```python
from build123d import *

# Parameters (mm, degrees)
SKETCH1_W           = 44
SKETCH1_H           = 72
BOSS_EXTRUDE1_DEPTH = 3
SKETCH2_W           = 44
SKETCH2_H           = 72
SKETCH2_W_2         = 40
SKETCH2_H_2         = 68
BOSS_EXTRUDE2_DEPTH = 34
SKETCH3_W           = 68
SKETCH3_H           = 109
SKETCH3_W_2         = 44
SKETCH3_H_2         = 72
BOSS_EXTRUDE3_DEPTH = 3
CHAMFER1_SIZE       = 0.528980942
CHAMFER1_SIZE_2     = 3


with BuildPart() as part:
    # Sketch1 → Boss-Extrude1 (new body)
    with BuildSketch(Plane(origin=(0, 0, 0), x_dir=(1, 0, 0), z_dir=(0, 1, 0))):
        with Locations((22, 36)):
            Rectangle(SKETCH1_W, SKETCH1_H)
    extrude(amount=BOSS_EXTRUDE1_DEPTH)

    # Sketch2 → Boss-Extrude2 (add)
    with BuildSketch(Plane(origin=(0, 3, 0), x_dir=(1, 0, 0), z_dir=(0, 1, 0))):
        with Locations((22, 36)):
            Rectangle(SKETCH2_W, SKETCH2_H)
        with Locations((22, 36)):
            Rectangle(SKETCH2_W_2, SKETCH2_H_2, mode=Mode.SUBTRACT)
    extrude(amount=BOSS_EXTRUDE2_DEPTH)

    # Sketch3 → Boss-Extrude3 (add)
    with BuildSketch(Plane(origin=(0, 24.3, 0), x_dir=(1, 0, 0), z_dir=(0, 1, 0))):
        with Locations((22, 36)):
            Rectangle(SKETCH3_W, SKETCH3_H)
        with Locations((22, 36)):
            Rectangle(SKETCH3_W_2, SKETCH3_H_2, mode=Mode.SUBTRACT)
        with BuildLine():
            Line((20.7, -3.5), (23.3, -3.5))
            ThreePointArc((23.3, -3.5), (25.6, -5.8), (23.3, -8.1))
            Line((23.3, -8.1), (20.7, -8.1))
            ThreePointArc((20.7, -8.1), (18.4, -5.8), (20.7, -3.5))
        make_face(mode=Mode.SUBTRACT)
        with BuildLine():
            Line((20.7, 75.5), (23.3, 75.5))
            ThreePointArc((23.3, 75.5), (25.6, 77.8), (23.3, 80.1))
            Line((23.3, 80.1), (20.7, 80.1))
            ThreePointArc((20.7, 80.1), (18.4, 77.8), (20.7, 75.5))
        make_face(mode=Mode.SUBTRACT)
    extrude(amount=BOSS_EXTRUDE3_DEPTH)

    # Chamfer1
    # the kernel refuses this chamfer: 3, 0.528980942 mm, written as the material it takes off along each edge
    with BuildSketch(Plane(origin=(-19.795616389, 27.3, -90.5), x_dir=(0, 0.21013876076743068, 0.9776715712462589), z_dir=(1, 0, 0)), Plane(origin=(63.795616389, 27.3, 18.5), x_dir=(0, 0.21013876076743068, -0.9776715712462589), z_dir=(-1, 0, 0))) as chamfer1_piece_1:
        Polygon((CHAMFER1_SIZE * 0.977671571478, CHAMFER1_SIZE * 0.210138760817), (-CHAMFER1_SIZE_2 * 0.210138760767, CHAMFER1_SIZE_2 * 0.977671571246), (0, 0), align=None)
    extrude(amount=83.591232779, mode=Mode.SUBTRACT)
    with BuildSketch(Plane(origin=(-12, 27.3, 26.295616389), x_dir=(0.9776715712462593, 0.21013876076742874, 0), z_dir=(0, 0, -1)), Plane(origin=(56, 27.3, -98.295616389), x_dir=(-0.9776715712462594, 0.21013876076742807, 0), z_dir=(0, 0, 1))) as chamfer1_piece_2:
        Polygon((CHAMFER1_SIZE * 0.977671571478, CHAMFER1_SIZE * 0.210138760817), (-CHAMFER1_SIZE_2 * 0.210138760767, CHAMFER1_SIZE_2 * 0.977671571246), (0, 0), align=None)
    extrude(amount=124.591232779, mode=Mode.SUBTRACT)


solid = part.part
```
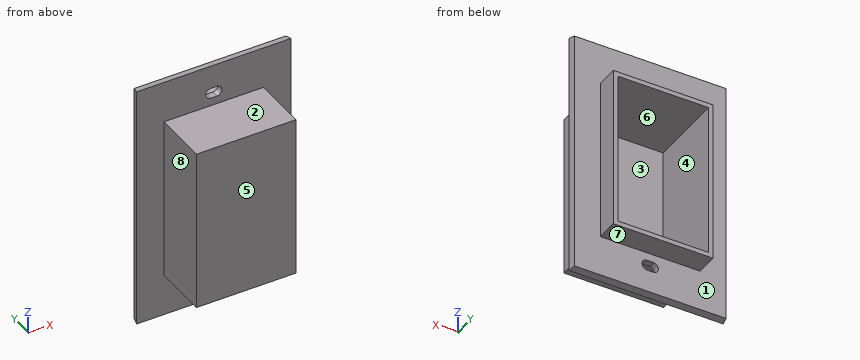
Read the model definition and answer for the solid it produces. Units are mm, in the model's axes. Face numbers are marked on the shaded views. A direction names the side the tool comes from. Give positions to 0.01 mm unless a question says otherwise; leave off trailing zeros. Loops run counter-clockwise (first coordinate to the right, second up) from the corner with the lowest first, then second, coordinate; pieces in that order, holes last.
Item 1: The part is cut by section B-B (y = 22.5). Write down the section's boundary in (x, z).
Item 2: The part is cut by section D-D (z = -81.5). Write down the section's boundary in (x, y), and give its area (3 significant figures).
Item 3: For the marked faces 5, 6, 7 and 8, determine the directions among +Z, -Z, +X, -X, +Y, -Y from which every point of the face is accessible in a straight line to the end or side of a thin tool.
Item 4: Find the intervals of material crossed by line 1 along X through (y, z) = (18, -3); line 2 along Z through (x, y) = (4.5, 7); line 3 along Y through (x, z) = (-9, -33.5), in increasing order.
Item 5: The part is cut by section C-C (z = -52). Write down the section's boundary in (x, y).
Item 6: The mould has two halves that part along Z. Classify the marked faces 1, 2, 3 and 4: released by +Z, released by -Z, zero draft, split by the parting line, or undercut.
Item 7: Each of these flat-tipped pins is pushed along its axis until it touches: pin 1 Ø0.8 at (x, y) = (22, 26) entering from -Z; pin 2 Ø20 at (x, z) = (31.5, -49.5) entering from +Y; pin 3 Ø12 at (y, z) = (16.5, -8.5) entering from -X. Where does it stop, or does it pass through?
Item 8: The part is cut by section A-A (z = 5.8). Write down the section's boundary in (x, y).
Taken from the geometry:
1. outline: (0, -72) - (44, -72) - (44, 0) - (0, 0) - close; hole (2, -70) - (42, -70) - (42, -2) - (2, -2) - close
2. outline: (-12, 24.3) - (56, 24.3) - (55.47, 27.3) - (-11.47, 27.3) - close
2. area: 202 mm2
3. face 5: +Z, -Z, +X, -X, -Y
3. face 6: +Y
3. face 7: -Z, +X, -X, +Y
3. face 8: +Z, -Z, -X, -Y
4. line 1: x = 0 to 2, 42 to 44
4. line 2: z = -72 to -70, -2 to 0
4. line 3: y = 24.3 to 27.3
5. outline: (-12, 24.3) - (0, 24.3) - (0, 0) - (44, 0) - (44, 24.3) - (56, 24.3) - (55.47, 27.3) - (44, 27.3) - (44, 37) - (42, 37) - (42, 3) - (2, 3) - (2, 37) - (0, 37) - (0, 27.3) - (-11.47, 27.3) - close
6. face 1: zero draft
6. face 2: released by +Z
6. face 3: undercut
6. face 4: undercut
7. pin 1: stops at z = -90.27
7. pin 2: stops at y = 3
7. pin 3: stops at x = 0
8. outline: (-12, 24.3) - (18.4, 24.3) - (18.4, 27.3) - (-11.47, 27.3) - close; (25.6, 24.3) - (56, 24.3) - (55.47, 27.3) - (25.6, 27.3) - close
